CAD build for the part. Positions are in the model's coordinates, mm. Coordinates: 2 decimals unless noted, no trailing zeros. Order: outer loops, then holes, each group sorted by start corner. A loop starts at its lowest first (then second) coordinate and runs counter-clockwise, first axis right, second up. Notation, with made-up numbers: M 19.5,-34 L 70.5,-34 A6 ccw 70.5,-26 Z; hole C -38,-8 d11. An arc over 180 degrees is marked long. Write item = value, one per line. Start each with the question number.
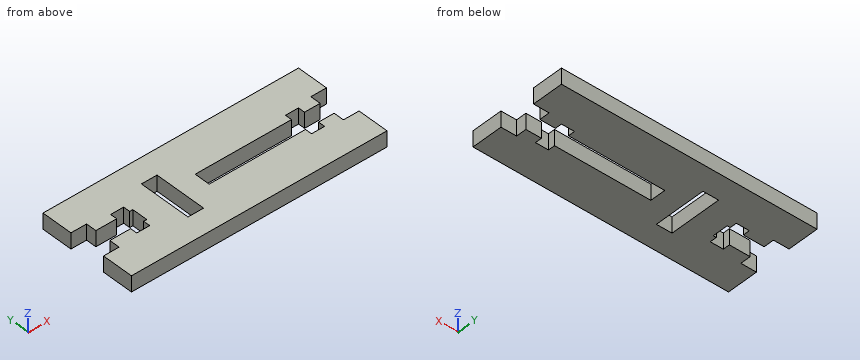
```python
from build123d import *

# Parameters (mm, degrees)
MODEL_W             = 3
MODEL_H             = 9.9999
BOSS_EXTRUDE1_DEPTH = 3


with BuildPart() as part:
    # Model → Boss-Extrude1 (new body)
    with BuildSketch(Plane.XY):
        Polygon((73.79, 50.5), (24.71, 50.5), (24.71, 44.5), (27.71, 44.5), (27.71, 42.5), (31.71, 42.5), (31.71, 43.8), (34.21, 43.8), (34.21, 42.5), (34.81, 42.5), (34.81, 39.5), (34.21, 39.5), (34.21, 38.2), (31.71, 38.2), (31.71, 39.5), (27.71, 39.5), (27.71, 37.5), (24.71, 37.5), (24.71, 31.5), (46.51, 31.5), (73.79, 31.5), (73.79, 37.5), (70.79, 37.5), (70.79, 39.5), (67.79, 39.5), (67.79, 38.2), (65.29, 38.2), (65.29, 39.5), (46.79, 39.5), (46.79, 42.5), (65.29, 42.5), (65.29, 43.8), (67.79, 43.8), (67.79, 42.5), (70.79, 42.5), (70.79, 44.5), (73.79, 44.5), align=None)
        with Locations((41.09, 41.00005)):
            Rectangle(MODEL_W, MODEL_H, mode=Mode.SUBTRACT)
    extrude(amount=BOSS_EXTRUDE1_DEPTH)


solid = part.part
```
1. Slice it at B-B (y = 36.5). Write the cut outline in (x, z).
2. Probe L1, parallel to Y at x = 61, z = 0.4; L2, parallel to X at y = 44.75, z = 2.3; L3, parallel to X at y = 40.75, z = 1.65. List the from-to ranges inside material, lowest first.
3. Slice it at A-A (x = 69). Write the cut outline in (y, z).
4. Flat gauge pins, fed straight in: pin 1 (1.4 mm diameter, centred on y = 38.5, z = 1.5, fed in from -X); pin 2 (1 mm diameter, centred on y = 43.5, z = 2, fed in from +X). Where does each tip first touch, or does it go through?
Calculated:
q1.outline = M 24.71,0 L 39.59,0 L 39.59,3 L 24.71,3 Z; M 42.59,0 L 73.79,0 L 73.79,3 L 42.59,3 Z
q2.L1 = 31.5 to 39.5, 42.5 to 50.5
q2.L2 = 24.71 to 39.59, 42.59 to 73.79
q2.L3 = 34.81 to 39.59, 42.59 to 46.79
q3.outline = M 31.5,0 L 39.5,0 L 39.5,3 L 31.5,3 Z; M 42.5,0 L 50.5,0 L 50.5,3 L 42.5,3 Z
q4.pin_1 = 27.71
q4.pin_2 = 70.79
